Build history of the part. All positions in model axes, mm. Face numbers are marked on the shaded views. Coordinates: 2 decimals unless noted, no trailing zeros. Loops run counter-clockwise (first coordinate to the right, second up) from the corner with the lowest first, then second, coordinate; pieces in that order, holes last.
(1) Slice it at D-D (x = -35.5). Give the cut face in (y, z), and give its area (3 significant figures).
(2) Slice it at B-B (z = 0.65). Give the cut face in (x, y).
(3) Slice it at A-A (x = -41.5). Give the cut face in (y, z), and give its area (3 significant figures).
(4) Two-plate mould, pull along X, no slides. Class the marked faces 1, 2 and 3: pulls with the +X half, pulls with the -X half, needs draft (parallel to the pull), parting line crosses it, or undercut.
(5) Wall check: L1, parallel to Z at x = -43, y = 14; L2, parallel to X at y = 6.5, z = 0.7; L3, parallel to X at y = 12, z = 4. Give the ranges that are in metal, low to high.
(6) Flat gauge pins, fed straight in: P1, Ø2, axis at x = -51, z = 0.5, coming from the -Y side; P2, Ø1.2, axis at y = 17, z = 1, coming from the -X side; P3, Ø3.5, axis at x = -41.52, y = -2.21, coming from the +Z side; P4, Ø1.8, axis at x = -51.52, y = -2.21, coming from the -Z side. Where does each tip first touch, or does it go through?
(7) Slice it at C-C (y = 14.5). Give the cut face in (x, z).
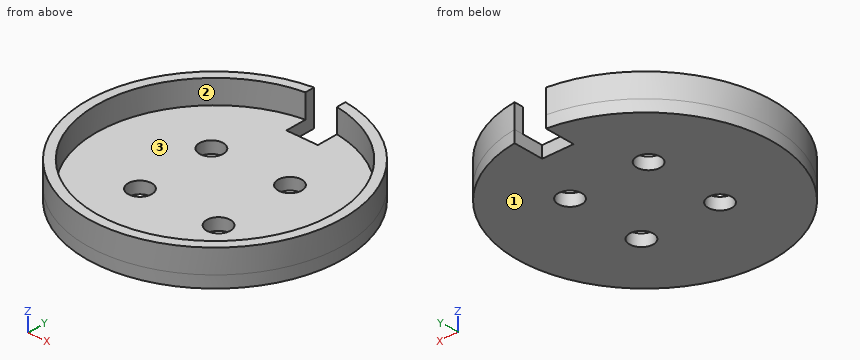
from build123d import *

# Parameters (mm, degrees)
CROQUIS1_R              = 1.5
SALIENTE_EXTRUIR1_DEPTH = 1.5
SALIENTE_EXTRUIR2_DEPTH = 3


with BuildPart() as part:
    # Croquis1 → Saliente-Extruir1 (new body)
    with BuildSketch(Plane.XY):
        with BuildLine():
            Line((-48.521455966, 14.990333384), (-48.521455966, 18.864023727))
            ThreePointArc((-48.521455966, 18.864023727), (-46.521455966, -13.412045444), (-44.521455966, 18.864023727))
            Line((-44.521455966, 18.864023727), (-44.521455966, 14.990333384))
            Line((-44.521455966, 14.990333384), (-48.521455966, 14.990333384))
        make_face()
        with Locations((-41.521455966, -2.212045444)):
            Circle(CROQUIS1_R, mode=Mode.SUBTRACT)
        with Locations((-51.521455966, -2.212045444)):
            Circle(CROQUIS1_R, mode=Mode.SUBTRACT)
        with Locations((-51.521455966, 7.787954556)):
            Circle(CROQUIS1_R, mode=Mode.SUBTRACT)
        with Locations((-41.521455966, 7.787954556)):
            Circle(CROQUIS1_R, mode=Mode.SUBTRACT)
    extrude(amount=SALIENTE_EXTRUIR1_DEPTH)

    # Croquis2 → Saliente-Extruir2 (add)
    with BuildSketch(Plane.XY.offset(1.5)):
        with BuildLine():
            Line((-48.521455966, 18.864023727), (-48.521455966, 17.664023727))
            ThreePointArc((-48.521455966, 17.664023727), (-46.523016697, -12.202149494), (-44.521455966, 17.663814696))
            Line((-44.521455966, 17.663814696), (-44.521455966, 18.864023727))
            ThreePointArc((-44.521455966, 18.864023727), (-46.521455966, -13.412045444), (-48.521455966, 18.864023727))
        make_face()
    extrude(amount=SALIENTE_EXTRUIR2_DEPTH)


solid = part.part
Response values:
1. outline: (-9.09, 0) - (14.66, 0) - (14.66, 4.5) - (12.97, 4.5) - (12.97, 1.5) - (-7.38, 1.5) - (-7.38, 4.5) - (-9.09, 4.5) - close
1. area: 45.8 mm2
2. outline: (-48.52, 14.99) - (-48.52, 18.86) arc R16.2 ccw (long way) to (-44.52, 18.86) - (-44.52, 14.99) - close; hole circle Ø3 at (-51.52, -2.21); hole circle Ø3 at (-51.52, 7.79); hole circle Ø3 at (-41.52, -2.21); hole circle Ø3 at (-41.52, 7.79)
3. outline: (-12.61, 0) - (-3.71, 0) - (-3.71, 1.5) - (-11.34, 1.5) - (-11.34, 4.5) - (-12.61, 4.5) - close; (-0.71, 0) - (6.29, 0) - (6.29, 1.5) - (-0.71, 1.5) - close; (9.29, 0) - (18.19, 0) - (18.19, 4.5) - (16.93, 4.5) - (16.93, 1.5) - (9.29, 1.5) - close
3. area: 44.8 mm2
4. face 1: needs draft
4. face 2: undercut
4. face 3: undercut
5. L1: z = 0 to 1.5
5. L2: x = -62.29 to -52.29, -50.75 to -42.29, -40.75 to -30.75
5. L3: x = -59.85 to -58.37, -34.68 to -33.2
6. P1: stops at y = -13.03
6. P2: stops at x = -55.31
6. P3: stops at z = 1.5
6. P4: passes through
7. outline: (-57.71, 0) - (-35.33, 0) - (-35.33, 4.5) - (-37.14, 4.5) - (-37.14, 1.5) - (-55.91, 1.5) - (-55.91, 4.5) - (-57.71, 4.5) - close
